Check sheet for the modelled part. Datum: model origin and axes. Units: mm. Coordinates: 2 decimals unless noted, no trailing zeros. Loops run counter-clockwise (first coordinate to the right, second up) from the corner with the lowest first, then second, coordinate; pieces in that order, holes last. Notation, with made-up numbers: M 16,87 L 32,87 A17 ccw 32,112 Z; hole C 61,-3.5 d4. An arc over 180 degrees is marked long. Use CSV: the item, a comma, the result in double quotes. Start each with the question number.
(1) Go/stop test with flat-tipped pins: pin 1 Ø1.5 at (x, z) = (6.5, -3.5) entering from +Y; pin 2 Ø2 at (y, z) = (33.5, 1.5) entering from +X; pin 3 Ø6 at (x, z) = (1, 1.5) entering from +Y; pin 4 Ø1 at (x, y) = (6.5, 45) entering from +Z. Record where each tip stops, or that it passes through.
(2) Section check B-B on z = 0. Record the cut outline in (x, y).
(3) Section check C-C on y = 6.5. Record the cut outline in (x, z).
(4) Section check A-A on x = 0. Record the cut outline in (y, z).
(5) Scan lines: line 1 (X direction, y = 35, z = 0); line 2 (Z direction, x = -5, y = 4.5). Record each from-to range of solid material in increasing order.
(6) Draft check along Z on faces 1 (the flat face through (-8, 50, -1)), 2 (the cylindrical face through (6.466, 24.72, -2.681)), 3 (the cylindrical face through (-1.172, 11.586, 8.923)). Enter one of: pulls with the +Z half, pulls with the -Z half, needs draft (parallel to the pull), parting line crosses it, or undercut.
Solid Edge part; units mm, degrees
sketch "Sketch1" plane through (0, 0, 0) normal (0, -1, 0) x (1, 0, 0)
  circle A0 centre (0, 0) radius 9
  circle A1 centre (0, 0) radius 7
extrude "Protrusion1" add sketch "Sketch1" against normal blind 50
sketch "Sketch2" plane through (0, 0, 0) normal (0, 0, 1) x (1, 0, 0)
  arc A0 (-9, 23.5) -> (-7.5, 25) centre (-9, 25) ccw
  arc A1 (-7.5, 25) -> (-9, 26.5) centre (-9, 25) ccw
  line L0 (-9, 26.5) -> (-9, 23.5)
revolve "RevolvedCutout1" cut sketch "Sketch2" angle 360 about axis through (0, 52.7188, 0) along (0, -1, 0)
sketch "Sketch3" plane through (0, 0, 0) normal (1, 0, 0) x (0, 1, 0)
  line L0 (0, 7) -> (0, 7.8816)
  line L1 (0, 7.8816) -> (5, 7)
  line L2 (5, 7) -> (0, 7)
  line L3 (50, 7) -> (50, 7.8816)
  line L4 (50, 7.8816) -> (45, 7)
  line L5 (45, 7) -> (50, 7)
  dimension "D1" = 5
revolve "RevolvedCutout2" cut sketch "Sketch3" angle 360 about axis through (0, 0, 0) along (0, 1, 0)
Outcome:
1,pin 1,"stops at y = 50"
1,pin 2,"stops at x = 8.99"
1,pin 3,"passes through"
1,pin 4,"stops at z = 6.71"
2,outline,"M -9,0 L -7.88,0 L -7,5 L -7,45 L -7.88,50 L -9,50 L -9,26.5 A1.5 cw -9,23.5 Z; M 7,5 L 7.88,0 L 9,0 L 9,23.5 A1.5 cw 9,26.5 L 9,50 L 7.88,50 L 7,45 Z"
3,outline,"C 0,0 d18; hole C 0,0 d14"
4,outline,"M 0,-9 L 23.5,-9 A1.5 cw 26.5,-9 L 50,-9 L 50,-7.88 L 45,-7 L 5,-7 L 0,-7.88 Z; M 0,7.88 L 5,7 L 45,7 L 50,7.88 L 50,9 L 26.5,9 A1.5 cw 23.5,9 L 0,9 Z"
5,line 1,"x = -9 to -7, 7 to 9"
5,line 2,"z = -7.48 to -5.02, 5.02 to 7.48"
6,face 1,"needs draft"
6,face 2,"undercut"
6,face 3,"parting line crosses it"
